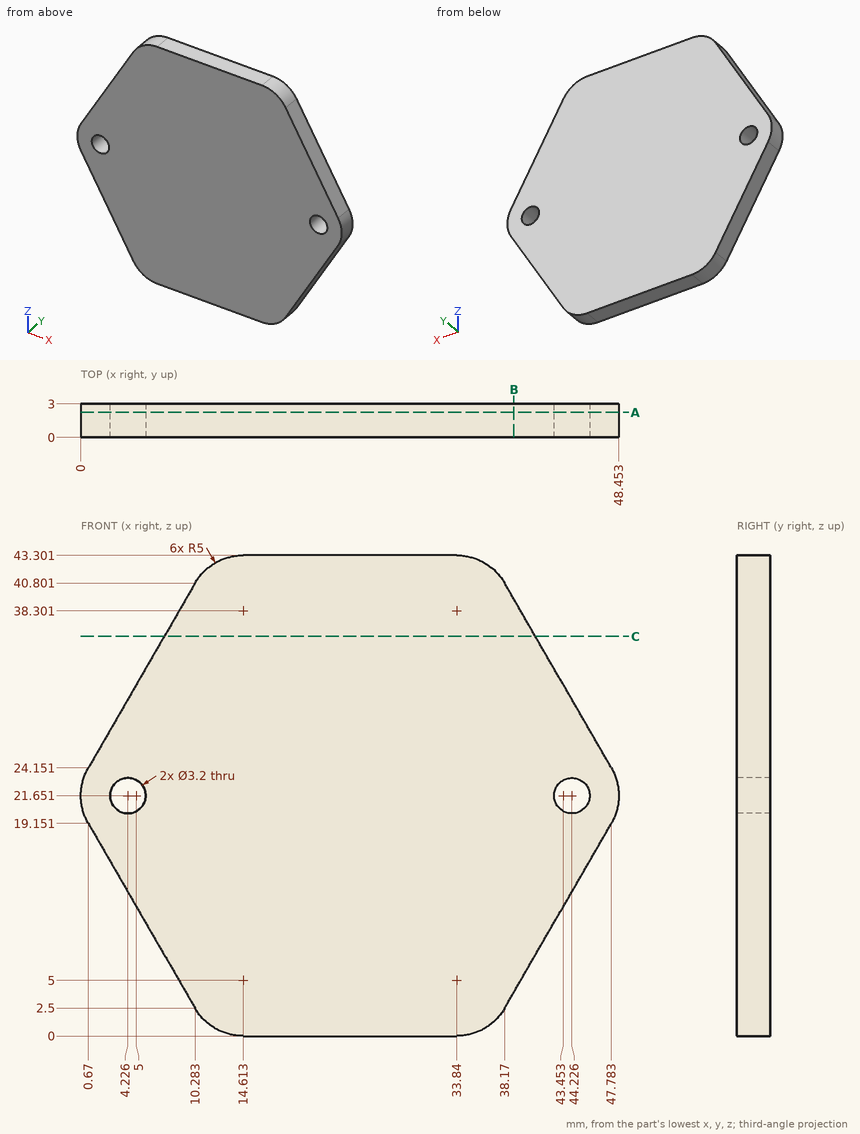
Part print with two shaded views. Sizes in mm from the minimum x, y, z corner. Give positions to 0.01 mm unless a question says otherwise; leave off trailing zeros. Write each loop counter-clockwise with the first axis right and the second up, starting at its lowest first coordinate (ties: lowest second). Pieces come first, ordered by that corner, then holes.
1) Cut at C-C on z = 36. Write the cut outline in (x, y), then the cut area to 3 significant figures.
Resolved:
outline: (7.51, 0) - (40.94, 0) - (40.94, 3) - (7.51, 3) - close
area: 100 mm2
2) Pin check, flat tips, straight feed: pin 1 (1.9 mm diameter, centred on x = 44.23, z = 21.65, fed in from -Y); pin 2 (6 mm diameter, centred on x = 8.5, z = 11, fed in from -Y); pin 3 (1 mm diameter, centred on x = 34.5, y = 1, fed in from -Z); pin 4 (1 mm diameter, centred on y = 1, z = 15.5, fed in from +X) (1 decimal). Stop position of each tip, or through.
Resolved:
pin 1: passes through
pin 2: stops at y = 0
pin 3: stops at z = 0
pin 4: stops at x = 46
3) Cut at A-A on y = 2.25. Write the cut outline in (x, z).
Resolved:
outline: (0.67, 19.15) - (10.28, 2.5) arc R5 ccw to (14.61, 0) - (33.84, 0) arc R5 ccw to (38.17, 2.5) - (47.78, 19.15) arc R5 ccw to (47.78, 24.15) - (38.17, 40.8) arc R5 ccw to (33.84, 43.3) - (14.61, 43.3) arc R5 ccw to (10.28, 40.8) - (0.67, 24.15) arc R5 ccw to start; hole circle Ø3.2 at (4.23, 21.65); hole circle Ø3.2 at (44.23, 21.65)
4) Cut at B-B on x = 39. Write the cut outline in (y, z), then the cut area to 3 significant figures.
Resolved:
outline: (0, 3.94) - (3, 3.94) - (3, 39.36) - (0, 39.36) - close
area: 106 mm2
5) Probe L1, parallel to X at y = 2.35, z = 21 (1 decimal); L2, parallel to Z at x = 43, y = 2.25 (1 decimal); L3, parallel to Z at x = 44, y = 0.7 (1 decimal). List the from-to ranges inside material, lowest first.
Resolved:
L1: x = 0 to 2.8, 5.7 to 42.8, 45.7 to 48.4
L2: z = 10.9 to 20.6, 22.7 to 32.4
L3: z = 12.6 to 20.1, 23.2 to 30.7
